The listing builds one solid part. Answer for the finished solid, in the listing's coordinates (mm). A direction names the side the tool comes from. Give positions to 0.01 mm unless a question says otherwise; leave off trailing zeros. Loops run counter-clockwise (first coordinate to the right, second up) from the corner with the lowest first, then second, coordinate; pieces in that order, holes last. Notation, with made-up numbers: (71, -36.75) - (75, -36.75) arc R18 cw to (75, -12.75) - close; hole circle Ø10 at (15.25, 39). An arc over 180 degrees is marked (long way). Write item = value, one per line. Start each with the question number.
1) The part is cut by section C-C on y = 24. Write down the section's boundary in (x, z), plus the area to 3 significant figures.
2) Consider probe 1 along Y at (x, z) = (-22, 2); probe 2 along X at (y, z) = (4, 0.9). Determine where each line is inside the solid, lowest interval first.
3) The part is cut by section B-B on x = 23.5. Write down the section's boundary in (y, z), plus the area to 3 significant figures.
4) The mould has two halves that part along Y. Classify faces 1 (the flat face through (-45, -32, 1)), 2 (the flat face through (56, 0, 1)), 3 (the flat face through (-58, 22.5, 1)), 4 (the flat face through (-58, -7.5, 1)): +Y half, -Y half, draft (parallel to the pull), parting line (faces both ways), or undercut.
5) Which of the six approach directions +Z, -Z, +X, -X, +Y, -Y give full straight-line access (tool end or side, diameter ignored) to faces 5 (the flat face through (50, -30, 1)), 6 (the flat face through (25, -32, 1)), 7 (the flat face through (56, 26, 1)), 8 (the flat face through (-51, -30, 1))?
6) Flat-ended cylindrical pins translate along their axes: P1, Ø0.9, axis at y = -24.5, z = 2, coming from the -X side; P2, Ø1.5, axis at x = -57.5, z = 2, coming from the -Y side; P3, Ø1.5, axis at x = -58, z = 1.5, coming from the +Y side. Find the tip coordinate at first contact, or state that the pin passes through.
from build123d import *

# Parameters (mm, degrees)
SKETCH2_W           = 3
SKETCH2_H           = 15
SKETCH2_W_2         = 112
SKETCH2_H_2         = 60
SKETCH2_W_3         = 20
SKETCH2_H_3         = 3
BOSS_EXTRUDE1_DEPTH = 3


with BuildPart() as part:
    # Sketch2 → Boss-Extrude1 (new body)
    with BuildSketch(Plane.XY):
        with Locations((-57.5, 15)):
            Rectangle(SKETCH2_W, SKETCH2_H)
        with Locations((-57.5, -15)):
            Rectangle(SKETCH2_W, SKETCH2_H)
        Rectangle(SKETCH2_W_2, SKETCH2_H_2)
        with Locations((-35, -31.5)):
            Rectangle(SKETCH2_W_3, SKETCH2_H_3)
        with Locations((0, -31.5)):
            Rectangle(SKETCH2_W_3, SKETCH2_H_3)
        with Locations((35, -31.5)):
            Rectangle(SKETCH2_W_3, SKETCH2_H_3)
        with Locations((57.5, -15)):
            Rectangle(SKETCH2_W, SKETCH2_H)
        with Locations((57.5, 15)):
            Rectangle(SKETCH2_W, SKETCH2_H)
    extrude(amount=BOSS_EXTRUDE1_DEPTH)


solid = part.part
Answer below:
q1.outline = (-56, 0) - (56, 0) - (56, 3) - (-56, 3) - close
q1.area = 336 mm2
q2.probe_1 = -30 to 30
q2.probe_2 = -56 to 56
q3.outline = (-30, 0) - (30, 0) - (30, 3) - (-30, 3) - close
q3.area = 180 mm2
q4.face_1 = draft
q4.face_2 = undercut
q4.face_3 = +Y half
q4.face_4 = undercut
q5.face_5 = +Z, -Z, +X, -Y
q5.face_6 = +Z, -Z, -Y
q5.face_7 = +Z, -Z, +X, +Y
q5.face_8 = +Z, -Z, -X, -Y
q6.P1 = -56
q6.P2 = -22.5
q6.P3 = 22.5
